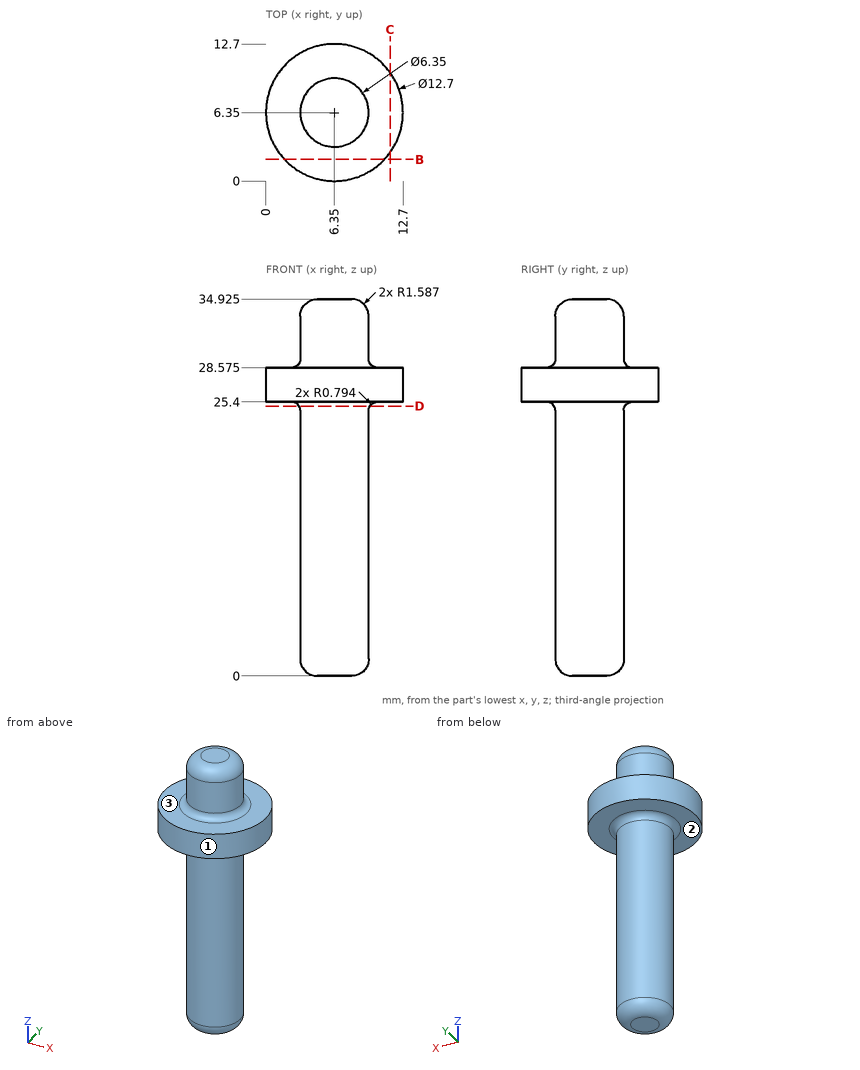
Can you work these out from the drawing? Everything is in mm from the part's minimum corner. A direction names the side the tool comes from. Coordinates: 2 decimals unless noted, no trailing zeros. Write each loop counter-clockwise with the first axis right and the second up, starting at its lowest first coordinate (ties: lowest second). Pieces come first, ordered by that corner, then holes. Notation, with made-up numbers: (67.25, 75) - (116.25, 75) arc R24 cw to (116.25, 87) - close; hole circle Ø2 at (41, 72). An arc over 180 degrees is marked (long way). One line per item, written item: value.
1) Suppose I cut it at D-D on z = 25. Write out the boundary of the cut face in (x, y).
Model answer:
outline: circle Ø6.56 at (6.35, 6.35)
2) On a 3-axis mill with a long thin cutter (end or side, diameter ignored), from which of +Z, -Z, +X, -X, +Y, -Y can I reach the whole of each face in a straight line? I mean the marked faces 1, 2 and 3. Say none if no direction works.
Model answer:
face 1: +Z, -Z
face 2: -Z
face 3: +Z
3) Suppose I cut it at C-C on x = 11.5. Write out the boundary of the cut face in (y, z) (1 decimal).
Model answer:
outline: (2.6, 25.4) - (10.1, 25.4) - (10.1, 28.6) - (2.6, 28.6) - close
4) I'm going to push flat-ended pins straight in: P1, Ø6, axis at y = 2.5, z = 18, coming from the +X side; P2, Ø1.5, axis at y = 8.5, z = 11.5, coming from the -X side; P3, Ø6.5, axis at x = 8.5, y = 8.5, coming from the +Z side (1 decimal); P4, Ø3, axis at y = 7.5, z = 10, coming from the +X side (1 decimal). Where does each tip first touch, or does it pass through?
Model answer:
P1: stops at x = 9.41
P2: stops at x = 3.5
P3: stops at z = 34.9
P4: stops at x = 9.5
5) I need wall thicknesses on line 1 along Z through (x, y) = (6.25, 12) (1 decimal); line 2 along Y through (x, z) = (6.5, 18). Which ranges of each line are inside material? Lowest first, please.
Model answer:
line 1: z = 25.4 to 28.6
line 2: y = 3.18 to 9.52
6) Suppose I cut it at B-B on y = 2. Write out the boundary of the cut face in (x, z) (1 decimal).
Model answer:
outline: (1.7, 25.4) - (11, 25.4) - (11, 28.6) - (1.7, 28.6) - close
